Job drawing, mm, ordinate dimensions from the low corner. One solid piece. Give positions to 0.01 mm unless a question says otherwise; leave off trailing zeros. Loops run counter-clockwise (first coordinate to the right, second up) from the corner with the lowest first, then second, coordinate; pieces in that order, holes last. Notation, with made-up numbers: (25, 0.25) - (45, 0.25) arc R36 ccw to (45, 35.25) - close; hole circle Ø7 at (49.5, -37). An arc over 180 degrees is marked (long way). Answer as CSV lines item,"result". Start each with the question number.
Item 1: Drill centre lines: L1, parallel to Y at x = 10.5, z = 68.7; L2, parallel to Z at x = 5, y = 15.25; L3, parallel to Z at x = 14.5, y = 17.5. Where is each one in solid material? Low to high. Write a range as from..to.
Item 2: Saw through at C-C on z = 10.5. Give the cut face in (x, y), plus the area to 3 significant figures.
Item 3: Saw through at B-B on x = 7. Give the cut face in (y, z), plus the area to 3 significant figures.
Item 4: Pin check, flat tips, straight feed: pin 1 (5 mm diameter, centred on x = 12.5, y = 6.5, fed in from -Z); pin 2 (1 mm diameter, centred on x = 18.5, y = 11.5, fed in from +Z); pin 3 (1 mm diameter, centred on x = 14, z = 27.5, fed in from -Y); pin 4 (2 mm diameter, centred on x = 2.5, z = 22, fed in from +Y). Stop position of each tip, or through.
Item 5: Saw through at D-D on y = 7.25. Give the cut face in (x, z), plus the area to 3 significant figures.
Item 6: Saw through at A-A on y = 16.25. Give the cut face in (x, z).
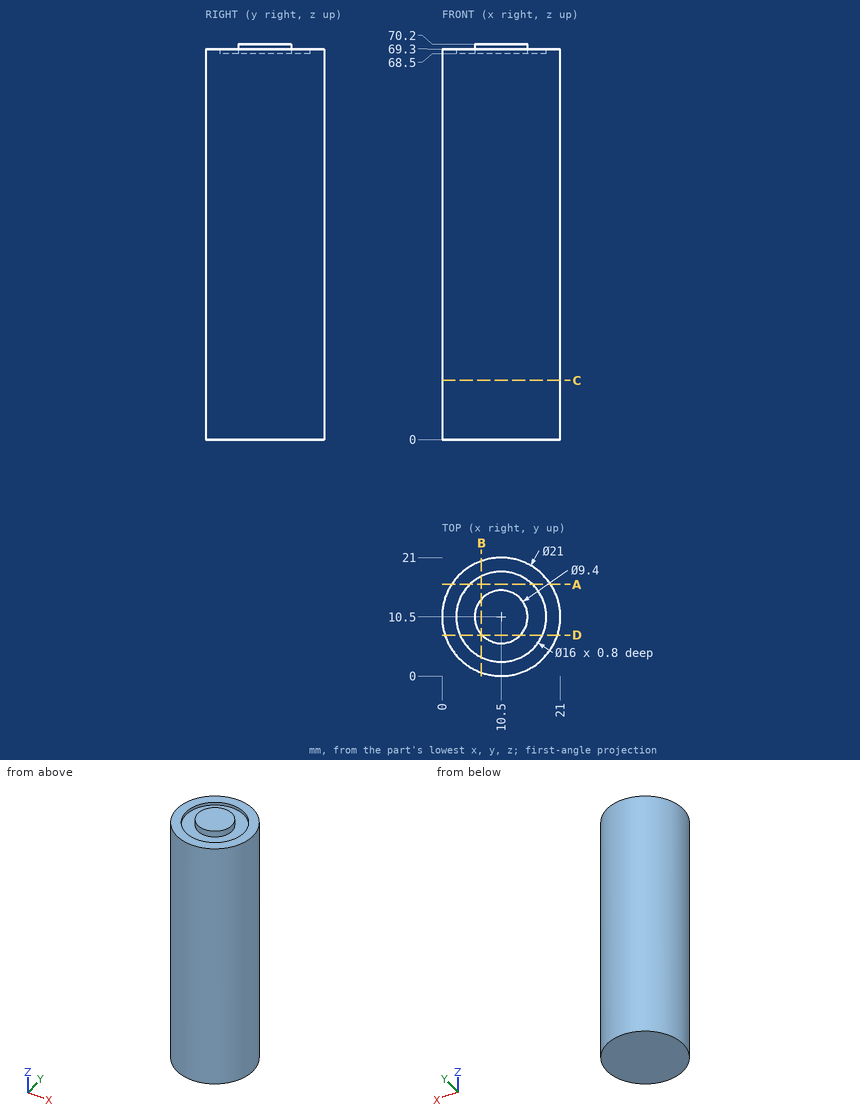
Responses:
1,L1,"0..2.5, 5.8..15.2, 18.5..21"
1,L2,"0..68.5"
1,L3,"0..69.3"
2,outline,"circle Ø21 at (10.5, 10.5)"
2,area,"346 mm2"
3,outline,"(0.6, 0) - (20.4, 0) - (20.4, 69.3) - (17.69, 69.3) - (17.69, 68.5) - (13.64, 68.5) - (13.64, 70.2) - (7.36, 70.2) - (7.36, 68.5) - (3.31, 68.5) - (3.31, 69.3) - (0.6, 69.3) - close"
3,area,"1,370 mm2"
4,pin 1,"z = 0"
4,pin 2,"z = 69.3"
4,pin 3,"y = 0.44"
4,pin 4,"y = 18.33"
5,outline,"(0.52, 0) - (20.48, 0) - (20.48, 69.3) - (17.81, 69.3) - (17.81, 68.5) - (13.9, 68.5) - (13.9, 70.2) - (7.1, 70.2) - (7.1, 68.5) - (3.19, 68.5) - (3.19, 69.3) - (0.52, 69.3) - close"
5,area,"1,380 mm2"
6,outline,"(1.71, 0) - (19.29, 0) - (19.29, 69.3) - (16.06, 69.3) - (16.06, 68.5) - (4.94, 68.5) - (4.94, 69.3) - (1.71, 69.3) - close"
